from build123d import *

# Parameters (mm, degrees)
SM_BASE_FLANGE_1_DEPTH = 25
SKETCH_6_R             = 1.5
CUT_EXTRUDE_1_DEPTH    = 37.728735344
SKETCH_7_R             = 1.5
CUT_EXTRUDE_2_DEPTH    = 35.942810419


# Sheet-metal steps are written as plain solids
with BuildPart() as part:
    # Sketch 1 → 基体-法兰1 (new body)
    with BuildSketch(Plane.XY):
        with BuildLine():
            Line((0, 20), (0, 4))
            ThreePointArc((0, 4), (1.171572875, 1.171572875), (4, 0))
            Line((4, 0), (20, 0))
            Line((20, 0), (20, 2))
            Line((20, 2), (4, 2))
            ThreePointArc((4, 2), (2.585786438, 2.585786438), (2, 4))
            Line((2, 4), (2, 20))
            Line((2, 20), (0, 20))
        make_face()
    extrude(amount=SM_BASE_FLANGE_1_DEPTH)

    # 草图6 → 切除-拉伸1 (cut, through all)
    with BuildSketch(Plane(origin=(0, 2, 0), x_dir=(1, 0, 0), z_dir=(0, 1, 0))):
        with Locations(Location((11, -5, 0), (0, 0, 270))):
            Circle(SKETCH_6_R)
        with Locations(Location((11, -20, 0), (0, 0, 90))):
            Circle(SKETCH_6_R)
        with BuildLine():
            Line((11, 0), (33.790991845, 0))
            Line((33.790991845, 0), (33.790991845, -25))
            Line((33.790991845, -25), (11, -25))
            ThreePointArc((11, -25), (14.535533906, -23.535533906), (16, -20))
            Line((16, -20), (16, -5))
            ThreePointArc((16, -5), (14.535533906, -1.464466094), (11, 0))
        make_face()
    extrude(amount=-CUT_EXTRUDE_1_DEPTH, mode=Mode.SUBTRACT)

    # 草图7 → 切除-拉伸2 (cut, through all)
    with BuildSketch(Plane(origin=(2, 0, 0), x_dir=(0, 0, -1), z_dir=(1, 0, 0))):
        with Locations(Location((-20, 11, 0), (0, 0, 90))):
            Circle(SKETCH_7_R)
        with Locations(Location((-5, 11, 0), (0, 0, 270))):
            Circle(SKETCH_7_R)
        with BuildLine():
            Line((-25, 11), (-25, 23.177465953))
            Line((-25, 23.177465953), (0, 23.177465953))
            Line((0, 23.177465953), (0, 11))
            ThreePointArc((0, 11), (-1.464466094, 14.535533906), (-5, 16))
            Line((-5, 16), (-20, 16))
            ThreePointArc((-20, 16), (-23.535533906, 14.535533906), (-25, 11))
        make_face()
    extrude(amount=-CUT_EXTRUDE_2_DEPTH, mode=Mode.SUBTRACT)


solid = part.part
Could you check a few things on this model? Use its own coordinates, in mm. A direction names the side the tool comes from. Coordinates: 2 decimals unless noted, no trailing zeros. Write each loop counter-clockwise with the first axis right and the second up, starting at its lowest first coordinate (ties: lowest second). Pieces come first, ordered by that corner, then holes. Notation, with made-up numbers: (54, 35) - (61, 35) arc R20 cw to (61, 65) - close; hole circle Ø9 at (88, 3.25). An arc over 180 degrees is marked (long way). Put each result on its own line as item: value. Start each with the question number.
Q1. I want a section at A-A on z = 16.25. Write out the boundary of the cut face in (x, y).
Q2. Which directions (+Z, -Z, +X, -X, +Y, -Y) give clear straight access to the entire face, cutting with the end or side of a thin tool? Please do faces 4 (the cylindrical face through (15, 1, 2)), 5 (the flat face through (10, 2, 12)).
Q3. Please list where these lines run through material, in increasing order: L1, parallel to Z at x = 1, y = 11; L2, parallel to X at y = 0.5, z = 20; L3, parallel to X at y = 9.5, z = 20.5.
Q4. I'm going to push flat-ended pins straight in: P1, Ø9.5, axis at y = 12, z = 17, coming from the +X side; P2, Ø6, axis at x = 4.5, y = 8, coming from the +Z side; P3, Ø1.5, axis at x = 13, z = 3, coming from the +Y side; P4, Ø1, axis at y = 2, z = 9, coming from the -X side. Where does each tip first touch, or does it pass through?
Q5. I want a section at B-B on y = 12. Write out the boundary of the cut face in (x, z).
Q6. Thinking about a two-plate mould opening in Z: for faces 1 (the cylindrical face through (1, 15, 23)), 2 (the cylindrical face through (10.425, 1.014, 6.386)), 3 (the flat face through (0, 10, 12)), which applies, pulls with the +Z half, pulls with the -Z half, needs draft (parallel to the pull), parting line crosses it, or undercut?
Q7. I want a section at C-C on z = 5.75. Write out the boundary of the cut face in (x, y).
Checks:
1. outline: (0, 4) arc R4 ccw to (4, 0) - (16, 0) - (16, 2) - (4, 2) arc R2 cw to (2, 4) - (2, 16) - (0, 16) - close
2. face 4: -Z, +X, +Y, -Y
2. face 5: +Z, -Z, +X, +Y
3. L1: 0 to 3.5, 6.5 to 18.5, 21.5 to 25
3. L2: 2.06 to 9.5, 12.5 to 16
3. L3: 0 to 2
4. P1: x = 2
4. P2: z = 25
4. P3: y = 2
4. P4: x = 0.29
5. outline: (0, 0.1) - (2, 0.1) - (2, 3.88) - (0, 3.88) - close; (0, 6.12) - (2, 6.12) - (2, 18.88) - (0, 18.88) - close; (0, 21.12) - (2, 21.12) - (2, 24.9) - (0, 24.9) - close
6. face 1: pulls with the +Z half
6. face 2: undercut
6. face 3: needs draft
7. outline: (0, 4) arc R4 ccw to (4, 0) - (9.7, 0) - (9.7, 2) - (4, 2) arc R2 cw to (2, 4) - (2, 9.7) - (0, 9.7) - close; (0, 12.3) - (2, 12.3) - (2, 16) - (0, 16) - close; (12.3, 0) - (16, 0) - (16, 2) - (12.3, 2) - close
